Read the model definition and answer for the solid it produces. Units are mm, in the model's axes. A direction names the side the tool comes from. Give positions to 0.01 mm unless a question says otherwise; leave off trailing zeros. Loops run counter-clockwise (first coordinate to the right, second up) from the corner with the lowest first, then second, coordinate; pieces in that order, holes last. Notation, with made-up numbers: (-33.5, 84.25) - (-14.5, 84.25) arc R31 cw to (-14.5, 118.25) - close; hole circle Ø5 at (-15.75, 53). An arc over 180 degrees is marked (long way). Put each result on its own line as item: value. Start each with the question number.
1. For faces 1 (the flat face through (2.824, 38, 10)), 2 (the flat face through (-7, 36.86, 10)), 3 (the flat face through (-19.176, 19, 10)), determine the directions among +Z, -Z, +X, -X, +Y, -Y from which every point of the face is accessible in a straight line to the end or side of a thin tool.
2. A cutting plane is placed at C-C, the plane z = 18.5. Determine the outline of the cut face in (x, y), plus the area to 3 significant figures.
3. Given pin 1 Ø8 at (y, z) = (4, 9.5) entering from +X; pin 2 Ø4 at (y, z) = (24.5, 8) entering from -X; pin 3 Ø4 at (x, z) = (-25, 16.5) entering from +Y, each flat-ended and moving along its own axis, determine where each tip first touches the part or whether it passes through.
4. A cutting plane is placed at B-B, the plane y = 6.5. Determine the outline of the cut face in (x, z).
5. A cutting plane is placed at D-D, the plane x = -43. Determine the outline of the cut face in (y, z), plus the area to 3 significant figures.
6. Consider L1, parallel to X at y = 37.5, z = 10; L2, parallel to Y at x = -22, z = 13.5; L3, parallel to X at y = 6, z = 2. Determine where each line is inside the solid, lowest interval first. Write a range as from..to.
7. A cutting plane is placed at A-A, the plane z = 10. Determine the outline of the cut face in (x, y).
8. For a pull along X with two mould halves and no side action, classify faces 4 (the flat face through (-18, 17, 0)), 5 (the cylindrical face through (-0.268, 37.874, 9.399)), 6 (the flat face through (-47.176, -2, 10)), 7 (the flat face through (-17.176, 17, 10)) as released by +X, released by -X, zero draft, split by the parting line, or undercut.
```python
from build123d import *

# Parameters (mm, degrees)
EXTRUDE_1_DEPTH     = 20
SKETCH_2_R          = 2
CUT_EXTRUDE_1_DEPTH = 20


with BuildPart() as part:
    # 草图1 → 凸台-拉伸1 (new body)
    with BuildSketch(Plane.XY):
        Polygon((-17.175607408, 38.860314389), (-7.175607408, 38.860314389), (2.824392592, 38.860314389), (2.824392592, 36.860314389), (-17.175607408, 36.860314389), (-17.175607408, -0.639685611), (-17.175607408, -2.639685611), (-47.175607408, -2.639685611), (-47.175607408, -0.639685611), (-19.175607408, -0.639685611), (-19.175607408, 38.860314389), align=None)
    extrude(amount=EXTRUDE_1_DEPTH)

    # 草图2 → 切除-拉伸1 (cut)
    with BuildSketch(Plane(origin=(0, 38.860314389, 0), x_dir=(1, 0, 0), z_dir=(0, 1, 0))):
        with Locations((-2.175607408, -10)):
            Circle(SKETCH_2_R)
    extrude(amount=-CUT_EXTRUDE_1_DEPTH, mode=Mode.SUBTRACT)


solid = part.part
```
Return value:
1. face 1: +Z, -Z, +X, +Y, -Y
1. face 2: +Z, -Z, +X, -Y
1. face 3: +Z, -Z, -X, +Y
2. outline: (-47.18, -2.64) - (-17.18, -2.64) - (-17.18, 36.86) - (2.82, 36.86) - (2.82, 38.86) - (-19.18, 38.86) - (-19.18, -0.64) - (-47.18, -0.64) - close
2. area: 179 mm2
3. pin 1: stops at x = -17.18
3. pin 2: stops at x = -19.18
3. pin 3: stops at y = -0.64
4. outline: (-19.18, 0) - (-17.18, 0) - (-17.18, 20) - (-19.18, 20) - close
5. outline: (-2.64, 0) - (-0.64, 0) - (-0.64, 20) - (-2.64, 20) - close
5. area: 40.0 mm2
6. L1: x = -19.18..-4.18, -0.18..2.82
6. L2: y = -2.64..-0.64
6. L3: x = -19.18..-17.18
7. outline: (-47.18, -2.64) - (-17.18, -2.64) - (-17.18, 36.86) - (-4.18, 36.86) - (-4.18, 38.86) - (-19.18, 38.86) - (-19.18, -0.64) - (-47.18, -0.64) - close; (-0.18, 36.86) - (2.82, 36.86) - (2.82, 38.86) - (-0.18, 38.86) - close
8. face 4: zero draft
8. face 5: undercut
8. face 6: released by -X
8. face 7: released by +X
